Can you work these out from the model? Positions are in its coordinate system, mm. Face numbers are marked on the shaded views. A direction names the side the tool comes from. Coordinates: 2 decimals unless noted, no trailing zeros. Order: outer loops, then holes, each group sorted by start corner. A loop starts at its lowest first (then second) coordinate and runs counter-clockwise, first axis right, second up. Notation, with made-up numbers: (25.25, 37) -> (55.25, 37) arc R16 cw to (55.25, 41) -> close; hole circle Ø8 at (40, 42.25). An arc over 180 degrees is marked (long way). Write item = value, one per line.
Autodesk Inventor part; units mm, degrees
ref_plane "YZ Plane" through (0, 0, 0) normal (1, 0, 0) x (0, 1, 0)
ref_plane "XZ Plane" through (0, 0, 0) normal (0, 1, 0) x (-1, 0, 0)
ref_plane "XY Plane" through (0, 0, 0) normal (0, 0, 1) x (1, 0, 0)
sketch "Sketch1" plane through (0, 0, 0) normal (0, 0, 1) x (1, 0, 0)
  line L0 (-17.5, 0) -> (17.5, 0) construction
  line L1 (0, 12.4072) -> (0, -12.4072) construction
  line L2 (-12.5394, 0) -> (-12.5394, 3)
  line L3 (-12.5394, 3) -> (-9.5394, 3)
  line L4 (0, 12.5394) -> (-3, 12.5394)
  line L5 (-3, 12.5394) -> (-3, 9.5394)
  circle A0 centre (0, 0) radius 10 construction
  circle A1 centre (0, 0) radius 17.5 construction
  arc A2 (-3, 9.5394) -> (-9.5394, 3) centre (0, 0) ccw
  arc A3 (-13.7055, 10.8817) -> (-17.5, 0) centre (0, 0) ccw
  line L6 (0, 0) -> (-12.3744, 12.3744) construction
  line L7 (0, 0) -> (17.5, 0) construction
  arc A4 (0, 17.5) -> (-10.8817, 13.7055) centre (0, 0) ccw
  arc A5 (-13.7055, 10.8817) -> (-10.8817, 13.7055) centre (-12.3744, 12.3744) ccw
  line L8 (12.5394, 3) -> (9.5394, 3)
  line L9 (3, 12.5394) -> (3, 9.5394)
  arc A6 (9.5394, 3) -> (3, 9.5394) centre (0, 0) ccw
  arc A7 (10.8817, 13.7055) -> (13.7055, 10.8817) centre (12.3744, 12.3744) ccw
  line L10 (12.5394, 0) -> (12.5394, 3)
  line L11 (0, 12.5394) -> (3, 12.5394)
  arc A8 (17.5, 0) -> (13.7055, 10.8817) centre (0, 0) ccw
  arc A9 (10.8817, 13.7055) -> (0, 17.5) centre (0, 0) ccw
  line L12 (-12.5394, 0) -> (-12.5394, -3)
  line L13 (-12.5394, -3) -> (-9.5394, -3)
  line L14 (-3, -12.5394) -> (-3, -9.5394)
  arc A10 (-9.5394, -3) -> (-3, -9.5394) centre (0, 0) ccw
  arc A11 (-17.5, 0) -> (-13.7055, -10.8817) centre (0, 0) ccw
  arc A12 (-10.8817, -13.7055) -> (-13.7055, -10.8817) centre (-12.3744, -12.3744) ccw
  line L15 (0, -12.5394) -> (-3, -12.5394)
  line L16 (3, -12.5394) -> (3, -9.5394)
  arc A13 (3, -9.5394) -> (9.5394, -3) centre (0, 0) ccw
  line L17 (12.5394, -3) -> (9.5394, -3)
  line L18 (0, -12.5394) -> (3, -12.5394)
  line L19 (12.5394, 0) -> (12.5394, -3)
  arc A14 (13.7055, -10.8817) -> (17.5, 0) centre (0, 0) ccw
  arc A15 (0, -17.5) -> (10.8817, -13.7055) centre (0, 0) ccw
  arc A16 (13.7055, -10.8817) -> (10.8817, -13.7055) centre (12.3744, -12.3744) ccw
  arc A17 (-10.8817, -13.7055) -> (0, -17.5) centre (0, 0) ccw
  point P0 (12.3744, 12.3744)
  point P1 (-12.3744, -12.3744)
  point P2 (12.3744, -12.3744)
  dimension "d2" = 35
  dimension "d0" = 3
  dimension "d1" = 20
  dimension "d3" = 135
  dimension "d4" = 2
extrude "Extrusion1" add sketch "Sketch1" along normal blind 24
properties part number "shaft_spacer"
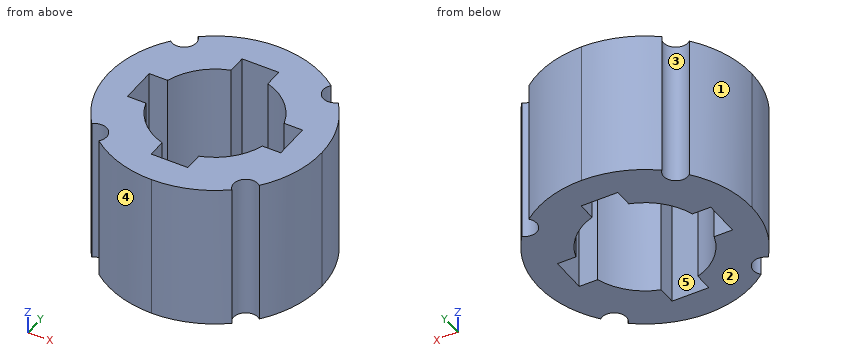
Item 1: I want a section at B-B, the plane x = 6.5. Please give me the cut outline in (y, z), plus the area to 3 significant figures.
A:
outline = (-16.25, 0) -> (-7.6, 0) -> (-7.6, 24) -> (-16.25, 24) -> close; (7.6, 0) -> (16.25, 0) -> (16.25, 24) -> (7.6, 24) -> close
area = 415 mm2
Item 2: I want a section at D-D, the plane x = 15. Please give me the cut outline in (y, z), plus the area to 3 significant figures.
A:
outline = (-9.01, 0) -> (9.01, 0) -> (9.01, 24) -> (-9.01, 24) -> close
area = 433 mm2
Item 3: If we mould it in two halves opening along X, with no side actions, what happens to the marked faces 1, 2 and 3? For each: pulls with the +X half, pulls with the -X half, needs draft (parallel to the pull), parting line crosses it, or undercut.
A:
face_1 = pulls with the -X half
face_2 = needs draft
face_3 = undercut
Item 4: I'm going to push flat-ended pins straight in: P1, Ø1.5, axis at x = 2.5, y = -13, coming from the -Z side; P2, Ø1.5, axis at x = 10.5, z = 16.5, coming from the -Y side; P3, Ø0.9, axis at x = -11.5, z = 17.5, coming from the -Y side; P4, Ø0.9, axis at x = -10.5, z = 11, coming from the +Y side. Where does each tip first touch, or does it pass through?
A:
P1 = 0
P2 = -14.53
P3 = -10.88
P4 = 14.33
Item 5: For the marked faces 4 and 5, which set-ups out of +Z, -Z, +X, -X, +Y, -Y let a thin tool reach every point of the face, with its end or its side?
A:
face_4 = +Z, -Z, -X, -Y
face_5 = +Z, -Z
Item 6: If I drill on probe 1 along Y at (x, z) = (-0.5, 14.5); probe 2 along Y at (x, z) = (-11.5, 10.5), over which ranges is the centre line in solid material (lowest first)?
A:
probe_1 = -17.49 to -12.54, 12.54 to 17.49
probe_2 = -10.58 to -3, 3 to 10.58
Item 7: I want a section at A-A, the plane z = 13.75. Please give me the cut outline in (x, y).
A:
outline = (-17.5, 0) arc R17.5 ccw to (-13.71, -10.88) arc R2 cw to (-10.88, -13.71) arc R17.5 ccw to (0, -17.5) arc R17.5 ccw to (10.88, -13.71) arc R2 cw to (13.71, -10.88) arc R17.5 ccw to (17.5, 0) arc R17.5 ccw to (13.71, 10.88) arc R2 cw to (10.88, 13.71) arc R17.5 ccw to (0, 17.5) arc R17.5 ccw to (-10.88, 13.71) arc R2 cw to (-13.71, 10.88) arc R17.5 ccw to start; hole (-12.54, -3) -> (-9.54, -3) arc R10 ccw to (-3, -9.54) -> (-3, -12.54) -> (3, -12.54) -> (3, -9.54) arc R10 ccw to (9.54, -3) -> (12.54, -3) -> (12.54, 3) -> (9.54, 3) arc R10 ccw to (3, 9.54) -> (3, 12.54) -> (-3, 12.54) -> (-3, 9.54) arc R10 ccw to (-9.54, 3) -> (-12.54, 3) -> close
Item 8: I want a section at C-C, the plane y = 1. Please give me the cut outline in (x, z).
A:
outline = (-17.47, 0) -> (-12.54, 0) -> (-12.54, 24) -> (-17.47, 24) -> close; (12.54, 0) -> (17.47, 0) -> (17.47, 24) -> (12.54, 24) -> close
